Geometry check sheet. Reference: drawing and pictorial views, mm from the part's lowest x, y, z. Give positions to 0.01 mm unless a question says otherwise; leave off trailing zeros. Order: outer loops, then holes, each group sorted by start corner. A loop starts at its lowest first (then second) coordinate and runs counter-clockwise, first axis right, second up. Notation, with made-up numbers: (45.25, 84.5) -> (57.25, 84.5) arc R31 ccw to (57.25, 122.5) -> close; hole circle Ø11 at (-36.75, 23). An arc over 180 degrees is marked (long way). Write each question's results on one line, items separated by ' | '.
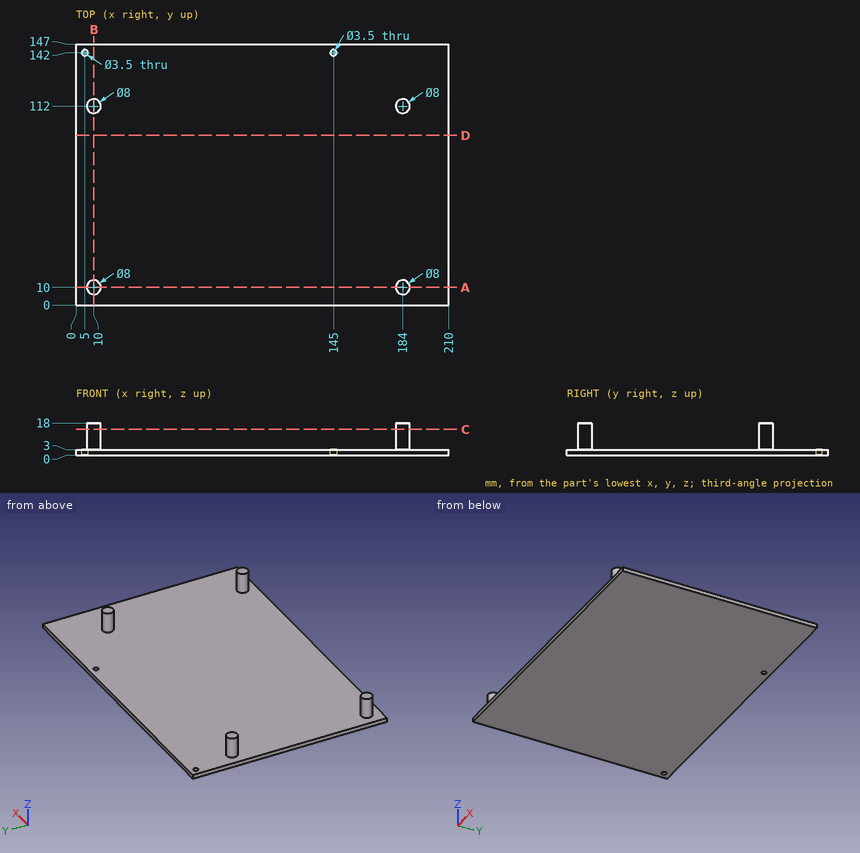
1. Section check D-D on y = 95.5. Record the cut outline in (x, z), then the cut area to 3 significant figures.
Verdict:
outline: (0, 0) -> (210, 0) -> (210, 3) -> (0, 3) -> close | area: 630 mm^2
2. Material ranges on probe 1 along X at (y, z) = (142, 1); probe 2 along Y at (x, z) = (5, 0.7); probe 3 along Z at (x, y) = (92, 44.5), recorded low to high. Write a range as from..to.
Verdict:
probe 1: x = 0..3.25, 6.75..143.25, 146.75..210 | probe 2: y = 0..140.25, 143.75..147 | probe 3: z = 0..3
3. Section check C-C on z = 14.5. Record the cut outline in (x, y), then the cut area to 3 significant figures.
Verdict:
outline: circle Ø8 at (10, 10); circle Ø8 at (10, 112); circle Ø8 at (184, 10); circle Ø8 at (184, 112) | area: 201 mm^2
4. Gauge pin test, flat ends, axial feed: pin 1 Ø4.5 at (x, y) = (5, 142) entering from +Z; pin 2 Ø2 at (x, y) = (145, 142) entering from +Z. Record the tip position at first contact, or that the pin passes through.
Verdict:
pin 1: stops at z = 3 | pin 2: passes through
5. Section check B-B on x = 10. Record the cut outline in (y, z).
Verdict:
outline: (0, 0) -> (147, 0) -> (147, 3) -> (116, 3) -> (116, 18) -> (108, 18) -> (108, 3) -> (14, 3) -> (14, 18) -> (6, 18) -> (6, 3) -> (0, 3) -> close
6. Section check A-A on y = 10. Record the cut outline in (x, z), then the cut area to 3 significant figures.
Verdict:
outline: (0, 0) -> (210, 0) -> (210, 3) -> (188, 3) -> (188, 18) -> (180, 18) -> (180, 3) -> (14, 3) -> (14, 18) -> (6, 18) -> (6, 3) -> (0, 3) -> close | area: 870 mm^2
